Print and shaded views of the part. All mm, measured from the part's lowest x, y and z. A direction names the side the tool comes from. Round coordinates to 2 decimals unless told otherwise and drop trailing zeros. Write each loop counter-clockwise with the first axis right and the second up, starting at its lowest first coordinate (ties: lowest second). Pieces come first, ordered by that corner, then holes. Notation, with made-up numbers: M 28.25,52.25 L 33.25,52.25 A30 ccw 33.25,85.25 Z; hole C -24,0 d10. An arc over 180 degrees is marked long. Write item = value, one per line. Start each with the question number.
Q1. Pull direction Z, two halves, no side cores. Call the marked faces 3, 4 and 5: released by +Z, released by -Z, zero draft, split by the parting line, or undercut.
Q2. Band-saw the part on D-D on z = 10. Write the cut outline in (x, y).
Q3. Band-saw the part on B-B on z = 27. Write the cut outline in (x, y).
Q4. Drop flat-ended pins along their axis: P1, Ø3.5, axis at y = 2, z = 6.5, coming from the -X side; P2, Ø3.5, axis at y = 3.5, z = 43.5, coming from the +X side (3 decimals); P3, Ø2, axis at y = 3.5, z = 6, coming from the +X side; P4, Ø20, axis at x = 27, z = 27, coming from the +Y side. Give the stop position or say it passes through.
Q5. Band-saw the part on A-A on x = 27. Write the cut outline in (y, z).
Q6. Band-saw the part on C-C on y = 1.25. Write the cut outline in (x, z).
Q7. Probe L1, parallel to X at y = 4.25, z = 9.5; L2, parallel to Z at x = 13, y = 4.75; L3, parallel to X at y = 1.75, z = 11. List the from-to ranges inside material, lowest first.
Q8. Tool access for the marked faces 1 and 2: list every direction of +Z, -Z, +X, -X, +Y, -Y with a clear straight run to the whole face (end or side of a thin tool).
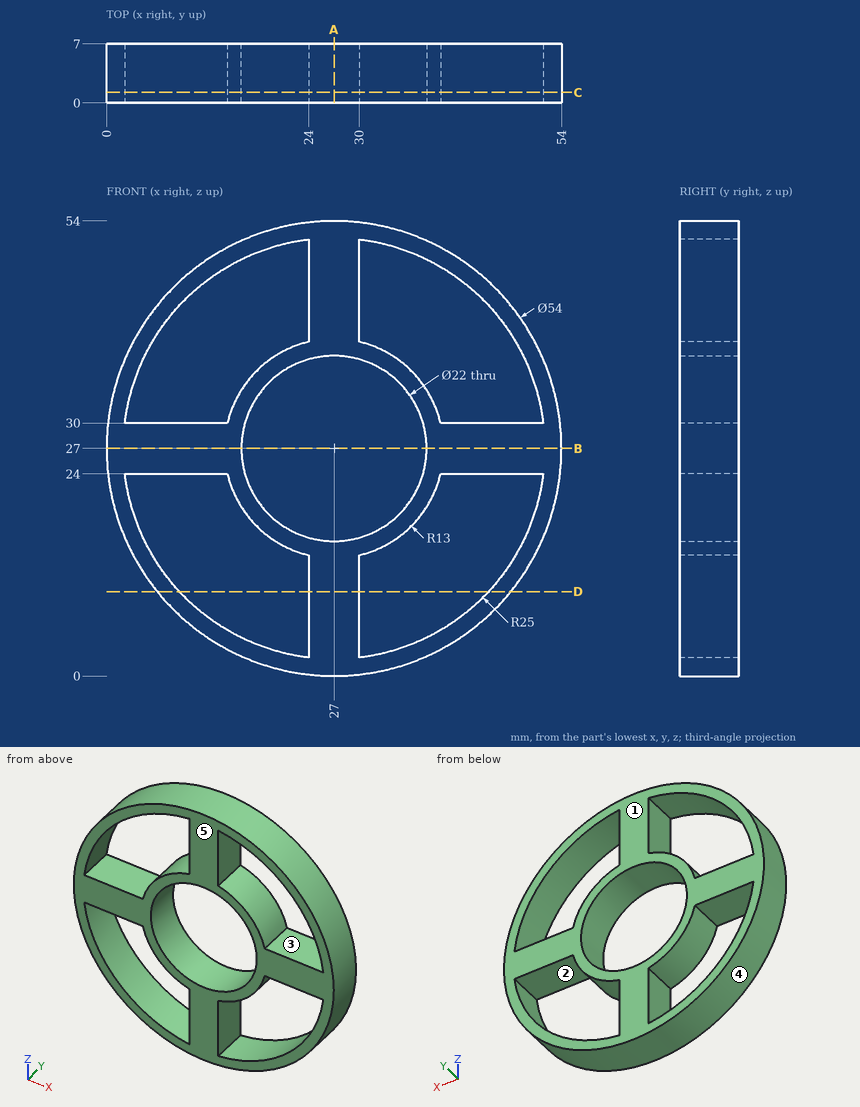
Conclusion:
q1.face_3 = undercut
q1.face_4 = split by the parting line
q1.face_5 = zero draft
q2.outline = M 6.02,0 L 8.67,0 L 8.67,7 L 6.02,7 Z; M 24,0 L 30,0 L 30,7 L 24,7 Z; M 45.33,0 L 47.98,0 L 47.98,7 L 45.33,7 Z
q3.outline = M 0,0 L 16,0 L 16,7 L 0,7 Z; M 38,0 L 54,0 L 54,7 L 38,7 Z
q4.P1 = 7.57
q4.P2 = 49.615
q4.P3 = 45.14
q4.P4 = through
q5.outline = M 0,0 L 7,0 L 7,16 L 0,16 Z; M 0,38 L 7,38 L 7,54 L 0,54 Z
q6.outline = C 27,27 d54; hole M 2.18,24 A25 ccw 24,2.18 L 24,14.35 A13 cw 14.35,24 Z; hole M 2.18,30 L 14.35,30 A13 cw 24,39.65 L 24,51.82 A25 ccw Z; hole C 27,27 d22; hole M 30,2.18 A25 ccw 51.82,24 L 39.65,24 A13 cw 30,14.35 Z; hole M 30,39.65 A13 cw 39.65,30 L 51.82,30 A25 ccw 30,51.82 Z
q7.L1 = 6.44 to 9.15, 24 to 30, 44.85 to 47.56
q7.L2 = 3.91 to 6.29, 24 to 30, 47.71 to 50.09
q7.L3 = 5.25 to 7.79, 24 to 30, 46.21 to 48.75
q8.face_1 = +Z, -Z, +X, -X, +Y
q8.face_2 = +Y, -Y
